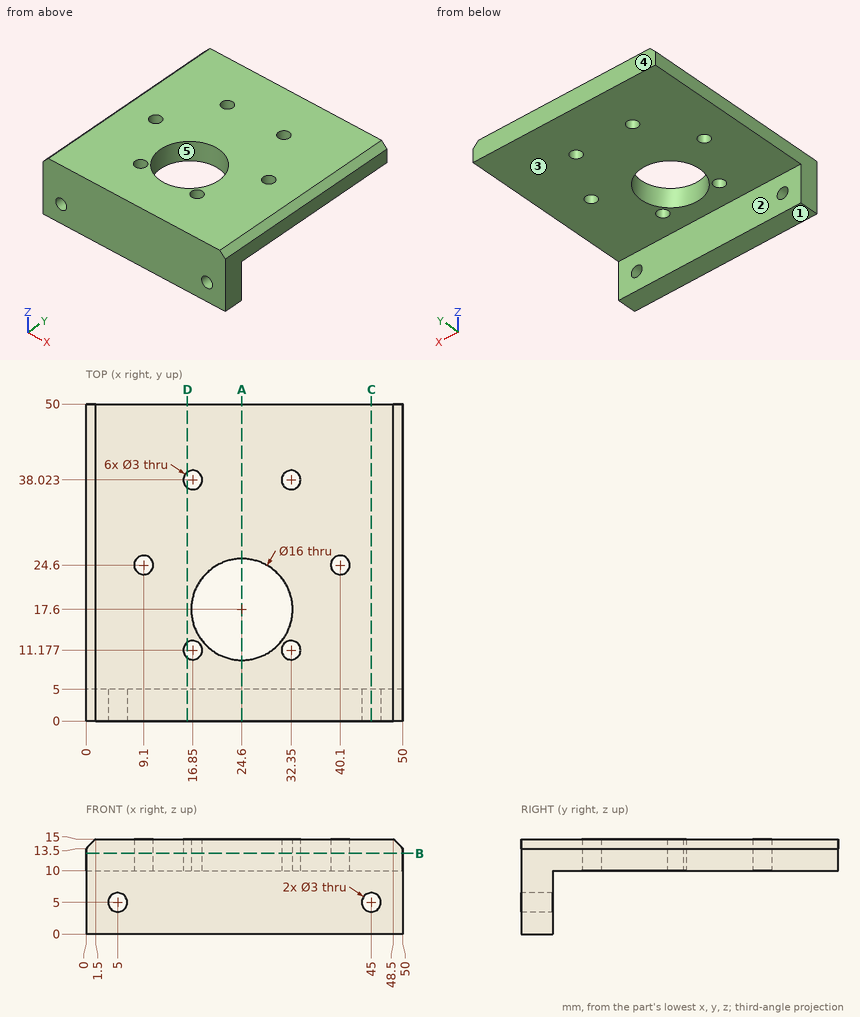
Source: three-view drawing plus pictorial views. Frame: mm from the lowest corner of the part. A direction names the side the tool comes from. Round coordinates to 2 decimals unless told otherwise and drop trailing zeros. Loops run counter-clockwise (first coordinate to the right, second up) from the corner with the lowest first, then second, coordinate; pieces in that order, holes last. Notation, with made-up numbers: (84.25, 44) -> (103.25, 44) arc R9 cw to (103.25, 57) -> close; hole circle Ø10 at (52, -33). An arc over 180 degrees is marked (long way). Use one line per item in the form item = value.
Item 1: Cut plane A-A on x = 24.6. Output: boundary loops of the cut face in (y, z).
Evaluation:
outline = (0, 0) -> (5, 0) -> (5, 10) -> (9.6, 10) -> (9.6, 15) -> (0, 15) -> close; (25.6, 10) -> (50, 10) -> (50, 15) -> (25.6, 15) -> close
Item 2: Draft query along Y for the marked faces 3, 4 and 5. Return one class per face: released by +Y, released by -Y, zero draft, split by the parting line, or undercut.
Evaluation:
face_3 = zero draft
face_4 = released by +Y
face_5 = undercut
Item 3: Cut plane D-D on x = 16. Output: boundary loops of the cut face in (y, z), then the cut area to 3 significant figures.
Evaluation:
outline = (0, 0) -> (5, 0) -> (5, 10) -> (9.94, 10) -> (9.94, 15) -> (0, 15) -> close; (12.41, 10) -> (36.79, 10) -> (36.79, 15) -> (12.41, 15) -> close; (39.26, 10) -> (50, 10) -> (50, 15) -> (39.26, 15) -> close
area = 275 mm2
Item 4: Cut plane B-B on z = 12.75. Output: boundary loops of the cut face in (x, y), then the cut area to 3 significant figures.
Evaluation:
outline = (0, 0) -> (50, 0) -> (50, 50) -> (0, 50) -> close; hole circle Ø3 at (9.1, 24.6); hole circle Ø3 at (16.85, 11.18); hole circle Ø3 at (16.85, 38.02); hole circle Ø16 at (24.6, 17.6); hole circle Ø3 at (32.35, 11.18); hole circle Ø3 at (32.35, 38.02); hole circle Ø3 at (40.1, 24.6)
area = 2,260 mm2
Item 5: Contact query for flat-ended pins moving along their axis: pin 1 Ø3 at (x, z) = (31.5, 5) entering from +Y; pin 2 Ø4 at (x, y) = (9, 20) entering from -Z; pin 3 Ø2.5 at (x, z) = (45, 5) entering from +Y. Output: stop coordinate, or through.
Evaluation:
pin_1 = 5
pin_2 = 10
pin_3 = through
Item 6: Access query for the marked faces 1 and 2. Directions: +Z, -Z, +X, -X, +Y, -Y. A direction counts if a zero-diameter tool reaches every point of the face in a straight line with its end or side. Return the directions, or none.
Evaluation:
face_1 = -Z, +X, -X, +Y, -Y
face_2 = -Z, +X, -X, +Y
Item 7: Cut plane C-C on x = 45. Output: boundary loops of the cut face in (y, z).
Evaluation:
outline = (0, 0) -> (5, 0) -> (5, 3.5) -> (0, 3.5) -> close; (0, 6.5) -> (5, 6.5) -> (5, 10) -> (50, 10) -> (50, 15) -> (0, 15) -> close
Item 8: Material intervals for probe 1 along Y at (x, z) = (40.1, 13.65); probe 2 along Z at (x, y) = (41, 33.5); probe 3 along X at (y, z) = (22.5, 12.25) (1 decimal), sorted ascending.
Evaluation:
probe_1 = 0 to 23.1, 26.1 to 50
probe_2 = 10 to 15
probe_3 = 0 to 18.3, 30.9 to 50
